```python
from build123d import *

# Parameters (mm, degrees)
F0_W     = 50.8
F0_H     = 4.7752
F0_H_2   = 4.7498
F0_W_2   = 0.8166841354
F0_H_3   = 19.05
F0_W_3   = 82.55
F1_DEPTH = 127


with BuildPart() as f1:
    # F0 (on Front) → F1 (new body)
    with BuildSketch(Plane.XZ):
        with Locations((85.725, 40.4876)):
            Rectangle(F0_W, F0_H)
        with Locations((85.725, 64.3001)):
            Rectangle(F0_W, F0_H_2)
        with Locations((111.5333420677, 52.4002)):
            Rectangle(F0_W_2, F0_H_3)
        with BuildLine():
            add(Edge.make_bspline(
                [(-41.275, 9.525), (-28.754702283, 46.6331869148), (-10.0444221635, 63.1745123066), (57.15, 61.9252)],
                knots=[0, 0, 0, 0, 111.5045361635, 111.5045361635, 111.5045361635, 111.5045361635], degree=3))
            Line((-41.275, 9.525), (41.275, 9.525))
            Line((41.275, 9.525), (41.275, 27.0002))
            ThreePointArc((41.275, 27.0002), (45.9246798487, 38.2255201513), (57.15, 42.8752))
            Line((57.15, 42.8752), (60.325, 42.8752))
            Line((60.325, 42.8752), (60.325, 61.9252))
            Line((60.325, 61.9252), (57.15, 61.9252))
        make_face()
        with Locations((85.725, 52.4002)):
            Rectangle(F0_W, F0_H_3)
        Rectangle(F0_W_3, F0_H_3)
    extrude(amount=F1_DEPTH)


solid = f1.part
```
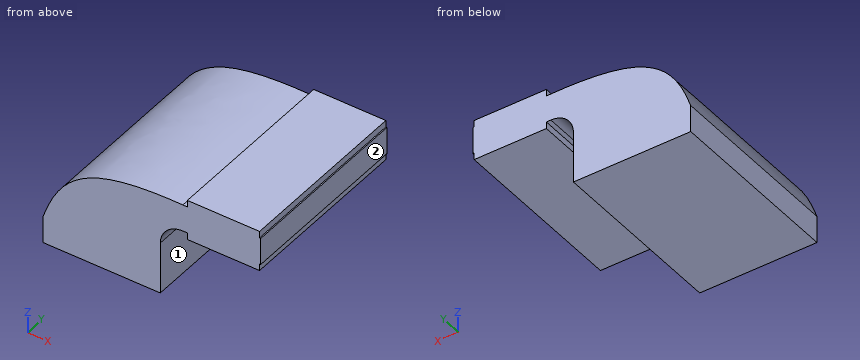
Work out the finished part from the listing and answer in its coordinate system (mm). Face numbers are marked on the shaded views. A direction names the side the tool comes from. Coordinates: 2 decimals unless noted, no trailing zeros. Write each loop counter-clockwise with the first axis right and the second up, starting at its lowest first coordinate (ties: lowest second). Pieces come first, ordered by that corner, then holes.
Q1. A cutting plane is placed at A-A, the plane z = 3. Give the vertices of the cut face in (x, y) (3 decimals).
Q2. Which of the six approach directions +Z, -Z, +X, -X, +Y, -Y give full straight-line access (tool end or side, diameter ignored) to the marked faces 1 and 2?
Q3. A cutting plane is placed at B-B, the plane x = 78.5. Give the vertices of the cut face in (y, z) (3 decimals), then the cut area to 3 significant figures.
Q4. Each of these flat-tipped pins is pushed along its axis until it touches: pin 1 Ø4 at (y, z) = (-39, 39.5) entering from -X; pin 2 Ø15 at (x, y) = (94.5, -89) entering from -Z; pin 3 Ø4 at (y, z) = (-53.5, 40.5) entering from +X (3 decimals); pin 4 Ø5 at (x, z) = (44.5, 30.5) entering from -Y. Where does it stop, or does it pass through?
Q5. Find the intervals of material crossed by line 1 (Z direction, x = 64, y = -37) (3 decimals); line 2 (X direction, y = -9, z = 6) (3 decimals); line 3 (Z direction, x = -22.5, y = -102.5) (3 decimals), in increasing order.
Findings below:
1. outline: (-41.275, -127) - (41.275, -127) - (41.275, 0) - (-41.275, 0) - close
2. face 1: -Z, +X, +Y, -Y
2. face 2: +Z, -Z, +X, +Y, -Y
3. outline: (-127, 38.1) - (0, 38.1) - (0, 66.675) - (-127, 66.675) - close
3. area: 3,630 mm2
4. pin 1: stops at x = -27.15
4. pin 2: stops at z = 38.1
4. pin 3: stops at x = 111.125
4. pin 4: passes through
5. line 1: z = 38.1 to 66.675
5. line 2: x = -41.275 to 41.275
5. line 3: z = -9.525 to 42.596
